from build123d import *

# Parameters (mm, degrees)
SKETCH068_R     = 19
PAD025_DEPTH    = 3
SKETCH069_R     = 4.5
POCKET042_DEPTH = 3.001
CHAMFER029_SIZE = 0.3
CHAMFER030_SIZE = 0.3
SKETCH070_R     = 8.25
POCKET043_DEPTH = 1


with BuildPart() as part:
    # Sketch068 → Pad025 (new body)
    with BuildSketch(Plane.XY):
        with Locations((0.140173, 0)):
            Circle(SKETCH068_R)
    extrude(amount=PAD025_DEPTH)

    # Sketch069 (on Face2 of Pad025) → Pocket042 (cut, through all)
    with BuildSketch(Plane(origin=(0, 0, 0), x_dir=(1, 0, 0), z_dir=(0, 0, -1))):
        Circle(SKETCH069_R)
    extrude(amount=-POCKET042_DEPTH, mode=Mode.SUBTRACT)

    # Chamfer029
    chamfer029_edges = [part.edges().sort_by_distance(p)[0] for p in [
        (-4.5, 0, 0),
        (-4.5, 0, 3),
    ]]
    chamfer(chamfer029_edges, length=CHAMFER029_SIZE)

    # Chamfer030
    chamfer030_edges = [part.edges().sort_by_distance(p)[0] for p in [
        (-18.859827, 0, 0),
        (-18.859827, 0, 3),
    ]]
    chamfer(chamfer030_edges, length=CHAMFER030_SIZE)

    # Sketch070 (on Face8 of Chamfer030) → Pocket043 (cut)
    with BuildSketch(Plane.XY.offset(3)):
        Circle(SKETCH070_R)
    extrude(amount=-POCKET043_DEPTH, mode=Mode.SUBTRACT)


solid = part.part
CAD build for the part. Positions are in the model's coordinates, mm. Coordinates: 2 decimals unless noted, no trailing zeros. Write each loop counter-clockwise with the first axis right and the second up, starting at its lowest first coordinate (ties: lowest second). Pieces come first, ordered by that corner, then holes. Notation, with made-up numbers: M 85.25,42 L 142.25,42 A12 ccw 142.25,54 Z; hole C 30.25,33.25 d4. An arc over 180 degrees is marked long. Return JSON: item names as keys, results as strings.
Item 1: Slice it at A-A, the plane y = 0. Write the cut outline in (x, z).
Findings below:
{"outline": "M -18.86,0.3 L -18.56,0 L -4.8,0 L -4.5,0.3 L -4.5,2 L -8.25,2 L -8.25,3 L -18.56,3 L -18.86,2.7 Z; M 4.5,0.3 L 4.8,0 L 18.84,0 L 19.14,0.3 L 19.14,2.7 L 18.84,3 L 8.25,3 L 8.25,2 L 4.5,2 Z"}
Item 2: Two-plate mould, pull along Y, no slides. Class faces 1 (the flat face through (8, -4, 3)), 2 (the cylindrical face through (7.62, -3.16, 2.51)), 3 (the flat face through (4, -4, 2)), 4 (the cylindrical face through (-3.979, -18.548, 1.483)): +Y half, -Y half, draft (parallel to the pull), parting line (faces both ways), or undercut.
Findings below:
{"face 1": "draft", "face 2": "undercut", "face 3": "undercut", "face 4": "parting line"}
Item 3: Drop flat-ended pins along their axis: pin 1 Ø5 at (x, y) = (2.5, -2.5) entering from +Z; pin 2 Ø1 at (y, z) = (12, 0.5) entering from -X. Give the stop position or say it passes through.
Findings below:
{"pin 1": "stops at z = 2", "pin 2": "stops at x = -14.98"}
Item 4: Slice it at B-B, the plane z = 0.9. Write the cut outline in (x, y).
Findings below:
{"outline": "C 0.14,0 d38; hole C 0,0 d9"}
Item 5: Probe line 1 (Y direction, x = 0, z = 2.45); line 2 (Y direction, x = 0, z = 1.55); line 3 (X direction, y = -1, z = 0.8). List the from-to ranges inside material, lowest first. Write a range as from..to.
Findings below:
{"line 1": "y = -19..-8.25, 8.25..19", "line 2": "y = -19..-4.5, 4.5..19", "line 3": "x = -18.83..-4.39, 4.39..19.11"}
